Geometry check sheet. Reference: drawing and pictorial views, mm from the part's lowest x, y, z. A direction names the side the tool comes from. Round coordinates to 2 decimals unless told otherwise and drop trailing zeros. Order: outer loops, then holes, each group sorted by start corner. A loop starts at its lowest first (then second) coordinate and runs counter-clockwise, first axis right, second up. Notation, with made-up numbers: (83, 56) -> (89, 56) arc R7 ccw to (89, 66) -> close; hole circle Ø5 at (33, 55). An arc over 180 degrees is marked (long way). Return JSON: item names as keys, results as strings. Group by question number.
1) Depth check by flat-ended pin: pin 1 (7.5 mm diameter, centred on x = 37, z = 11, fed in from +Y); pin 2 (0.8 mm diameter, centred on y = 2.5, z = 4, fed in from -X); pin 3 (6 mm diameter, centred on x = 14, z = 2.5, fed in from -Y); pin 4 (0.8 mm diameter, centred on y = 2, z = 7, fed in from +X). Enter the tip coordinate at first touch or a pass-through.
2) Section check B-B on z = 4.25. Enter the section's corners in (x, y), plus the area to 3 significant figures.
3) Draft check along X on the marked faces 3 and 4. Enter one of: pulls with the +X half, pulls with the -X half, needs draft (parallel to the pull), parting line crosses it, or undercut.
4) Scan lines: L1, parallel to X at y = 2.85, z = 8.75; L2, parallel to Y at x = 24.5, z = 4.5. Record each from-to range of solid material in increasing order.
5) Section check C-C on x = 13.5. Enter the section's corners in (y, z).
6) Section check A-A on y = 3.1. Enter the section's corners in (x, z).
7) Tool access check on the marked faces 1 and 2. Record the directions out of +Z, -Z, +X, -X, +Y, -Y that give a thin tool (end or side, any length) a straight path to the whole face; none if there is none.
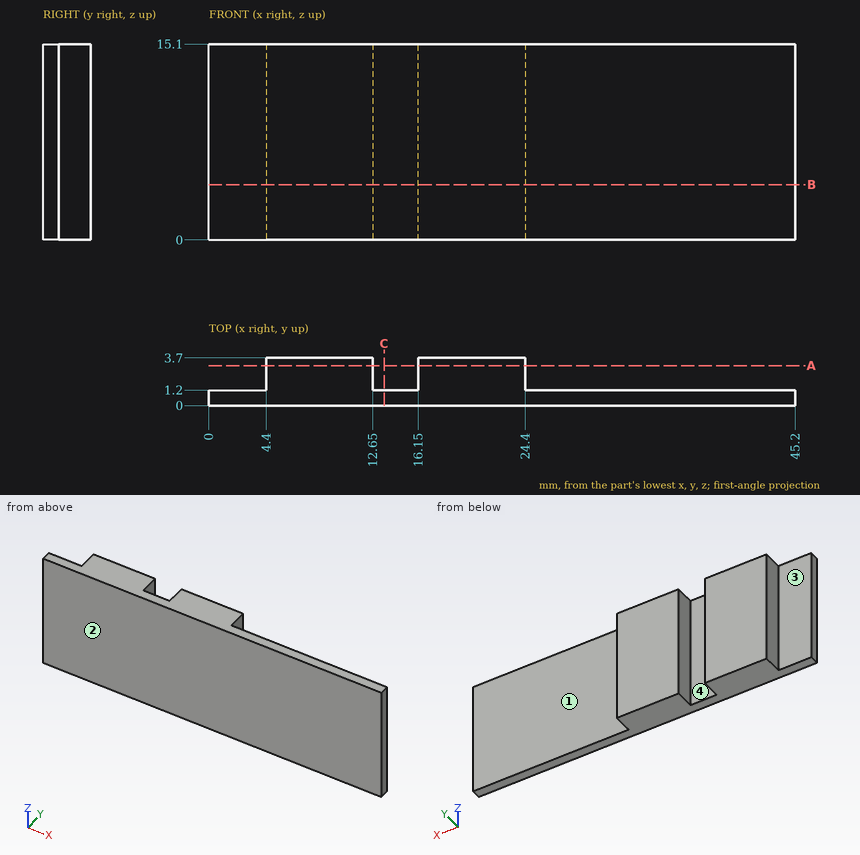
Check result:
{
 "1": {"pin 1": "y = 1.2", "pin 2": "x = 4.4", "pin 3": "y = 0", "pin 4": "x = 24.4"},
 "2": {"outline": "(0, 0) -> (45.2, 0) -> (45.2, 1.2) -> (24.4, 1.2) -> (24.4, 3.7) -> (16.15, 3.7) -> (16.15, 1.2) -> (12.65, 1.2) -> (12.65, 3.7) -> (4.4, 3.7) -> (4.4, 1.2) -> (0, 1.2) -> close", "area": "95.5 mm^2"},
 "3": {"face 3": "needs draft", "face 4": "undercut"},
 "4": {"L1": "4.4 to 12.65, 16.15 to 24.4", "L2": "0 to 1.2"},
 "5": {"outline": "(0, 0) -> (1.2, 0) -> (1.2, 15.1) -> (0, 15.1) -> close"},
 "6": {"outline": "(4.4, 0) -> (12.65, 0) -> (12.65, 15.1) -> (4.4, 15.1) -> close; (16.15, 0) -> (24.4, 0) -> (24.4, 15.1) -> (16.15, 15.1) -> close"},
 "7": {"face 1": "+Z, -Z, +X, +Y", "face 2": "+Z, -Z, +X, -X, -Y"}
}
